```python
from build123d import *

# Parameters (mm, degrees)
F_0_CLEARANCE_HOLE1_D     = 1.778
F_0_CLEARANCE_HOLE1_DEPTH = 19.05
F_0_CLEARANCE_HOLE1_TIP   = 0.53416509


with BuildPart() as part:
    # Sketch1 → Revolve1 (revolve)
    with BuildSketch(Plane(origin=(0, 0, 0), x_dir=(0, 0, -1), z_dir=(1, 0, 0)), mode=Mode.PRIVATE) as revolve1_sk:
        Polygon((0, 11), (0, 4.6), (2, 4.6), (2, 5.275), (8, 5.275), (8, 5.5), (17, 5.5), (17, 6.5), (2, 6.5), (2, 11), align=None)
    revolve(revolve1_sk.sketch.rotate(Axis((0, 0, 0), (0, 0, 1)), 90), axis=Axis((0, 0, 0), (0, 0, 1)))  # turned: the seam where the file's is

    # #0 Clearance Hole1
    with Locations(Plane(origin=(0, 0, -2), x_dir=(-1, 0, 0), z_dir=(0, 0, -1))):
        with Locations((0, 9.2718), (0, -9.2718)):
            Hole(F_0_CLEARANCE_HOLE1_D / 2, depth=F_0_CLEARANCE_HOLE1_DEPTH)
            with Locations((0, 0, -(F_0_CLEARANCE_HOLE1_DEPTH + F_0_CLEARANCE_HOLE1_TIP / 2))):  # 118° drill point
                Cone(0, F_0_CLEARANCE_HOLE1_D / 2, F_0_CLEARANCE_HOLE1_TIP, mode=Mode.SUBTRACT)


solid = part.part
```
Geometry: final body of the model. Coordinates: model frame, mm. A direction names the side the tool comes from. Coordinates: 2 decimals unless noted, no trailing zeros. Order: outer loops, then holes, each group sorted by start corner. A loop starts at its lowest first (then second) coordinate and runs counter-clockwise, first axis right, second up. Notation, with made-up numbers: (-9, 59) - (19, 59) arc R18 ccw to (19, 69) - close; hole circle Ø2 at (-31.75, 38). An arc over 180 degrees is marked (long way). Write each question's results on one line, items separated by ' | '.
1) Pin query (flat end, axial travel): pin 1 (4 mm diameter, centred on y = 2, z = -7.5, fed in from +X); pin 2 (2 mm diameter, centred on x = 0, y = 9.27, fed in from -Z); pin 3 (5 mm diameter, centred on y = -6, z = -5.5, fed in from -X); pin 4 (9 mm diameter, centred on x = 0, y = 0, fed in from +Z). Return the tip coordinate at first contact, or that it passes through.
Results list:
pin 1: x = 6.5 | pin 2: z = -2 | pin 3: x = -5.48 | pin 4: through
2) Pull-direction query (X, two-part tool) for faces 1 (the cylindrical face through (3.65, 2.8, -1.01)), 2 (the flat face through (-5, -3, -17)), 3 (the cylindrical face through (2.38, 10.74, -0.99)), 4 (the cylindrical face through (-0.19, -10.14, -0.99)); classes: pulls with the +X half, pulls with the -X half, needs draft (parallel to the pull), parting line crosses it, or undercut.
Results list:
face 1: undercut | face 2: needs draft | face 3: parting line crosses it | face 4: undercut
3) Section C-C, the plane x = 4. Return loops of the section in (y, z).
Results list:
outline: (-10.25, -2) - (-5.12, -2) - (-5.12, -17) - (-3.77, -17) - (-3.77, -8) - (-3.44, -8) - (-3.44, -2) - (-2.27, -2) - (-2.27, 0) - (-10.25, 0) - close; (2.27, -2) - (3.44, -2) - (3.44, -8) - (3.77, -8) - (3.77, -17) - (5.12, -17) - (5.12, -2) - (10.25, -2) - (10.25, 0) - (2.27, 0) - close
4) Section B-B, the plane y = -1. Return loops of the section in (x, z), plus the area to 3 significant figures.
Results list:
outline: (-10.95, -2) - (-6.42, -2) - (-6.42, -17) - (-5.41, -17) - (-5.41, -8) - (-5.18, -8) - (-5.18, -2) - (-4.49, -2) - (-4.49, 0) - (-10.95, 0) - close; (4.49, -2) - (5.18, -2) - (5.18, -8) - (5.41, -8) - (5.41, -17) - (6.42, -17) - (6.42, -2) - (10.95, -2) - (10.95, 0) - (4.49, 0) - close | area: 59.0 mm^2
5) Set-up query: faces 5 (the cylindrical face through (1.19, 5.37, -12.56)), 6 (the flat face through (0, 5, 0)). Return all of +Z, -Z, +X, -X, +Y, -Y with unobstructed straight access to the full face (end or side cutting, diameter ignored); none if empty.
Results list:
face 5: -Z | face 6: +Z, +X, -X, +Y, -Y
6) Line query: line 1 (Y direction, x = 0, z = -0.6); line 2 (Y direction, x = 0, z = -5.05) (3 decimals); line 3 (Z direction, x = 3.5, y = 9). Output: solid intervals per line, ascending. Write a range as from..to.
Results list:
line 1: -11..-10.16, -8.38..-4.6, 4.6..8.38, 10.16..11 | line 2: -6.5..-5.275, 5.275..6.5 | line 3: -2..0
7) Section A-A, the plane x = 0. Return loops of the section in (y, z) (3 decimals).
Results list:
outline: (-11, -2) - (-10.161, -2) - (-10.161, 0) - (-11, 0) - close; (-8.383, -2) - (-6.5, -2) - (-6.5, -17) - (-5.5, -17) - (-5.5, -8) - (-5.275, -8) - (-5.275, -2) - (-4.6, -2) - (-4.6, 0) - (-8.383, 0) - close; (4.6, -2) - (5.275, -2) - (5.275, -8) - (5.5, -8) - (5.5, -17) - (6.5, -17) - (6.5, -2) - (8.383, -2) - (8.383, 0) - (4.6, 0) - close; (10.161, -2) - (11, -2) - (11, 0) - (10.161, 0) - close
8) Section D-D, the plane z = -3. Return loops of the section in (x, y) (3 decimals), plus the area to 3 significant figures.
Results list:
outline: circle Ø13 at (0, 0); hole circle Ø10.55 at (0, 0) | area: 45.3 mm^2
